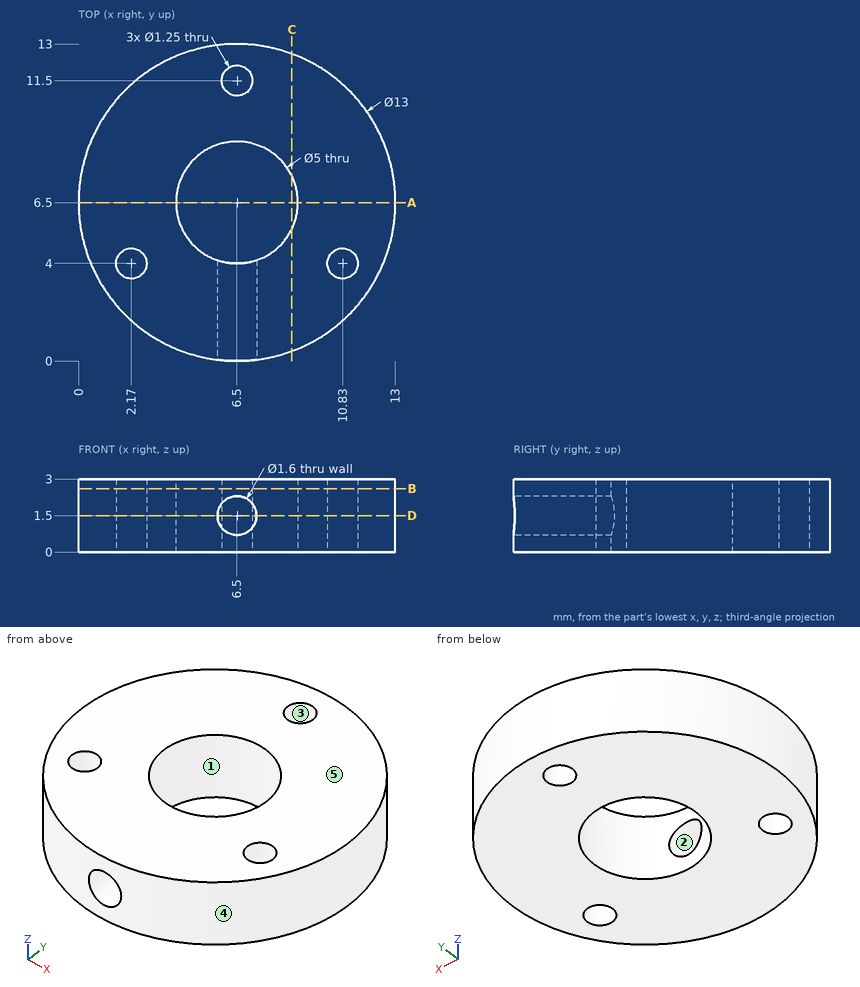
The figure shows three views and two pictorial views of one solid part (mm, origin at its lowest corner). Answer the questions. A direction names the side the tool comes from. Coordinates: 2 decimals unless noted, no trailing zeros. Order: outer loops, then holes, each group sorted by start corner. A loop starts at its lowest first (then second) coordinate and runs counter-clockwise, first axis right, second up.
Q1. Which of the six approach directions +Z, -Z, +X, -X, +Y, -Y give full straight-line access (tool end or side, diameter ignored) to the marked faces 1 and 2?
Q2. A cutting plane is placed at C-C, the plane x = 8.75. Write down the section's boundary in (y, z).
Q3. A cutting plane is placed at D-D, the plane z = 1.5. State how many separate pieces and enclosed holes the cut face has, and give its area (3 significant figures).
Q4. For a pull along X with two mould halves and no side action, classify the marked faces 3, 4 and 5 as pulls with the +X half, pulls with the -X half, needs draft (parallel to the pull), parting line crosses it, or undercut.
Q5. A cutting plane is placed at A-A, the plane y = 6.5. Write down the section's boundary in (x, z), and give its area (3 significant figures).
Q6. Consider line 1 (Y direction, x = 6.5, z = 0.8) (3 decimals); line 2 (X direction, y = 3.75, z = 1.7) (1 decimal); line 3 (X direction, y = 3.5, z = 0.45) (1 decimal). Determine where each line is inside the solid, lowest interval first.
Q7. A cutting plane is placed at B-B, the plane z = 2.6. Write down the section's boundary in (x, y) (3 decimals).
Answers follow:
1. face 1: +Z, -Z
1. face 2: -Y
2. outline: (0.4, 0) - (5.41, 0) - (5.41, 3) - (0.4, 3) - close; (7.59, 0) - (12.6, 0) - (12.6, 3) - (7.59, 3) - close
3. separate pieces: 1
3. enclosed holes: 3
3. area: 103 mm2
4. face 3: undercut
4. face 4: parting line crosses it
4. face 5: needs draft
5. outline: (0, 0) - (4, 0) - (4, 3) - (0, 3) - close; (9, 0) - (13, 0) - (13, 3) - (9, 3) - close
5. area: 24.0 mm2
6. line 1: y = 9 to 10.875, 12.125 to 13
6. line 2: x = 0.6 to 1.6, 2.7 to 5.7, 7.3 to 10.3, 11.4 to 12.4
6. line 3: x = 0.7 to 1.8, 2.5 to 10.5, 11.2 to 12.3
7. outline: circle Ø13 at (6.5, 6.5); hole circle Ø1.25 at (2.17, 4); hole circle Ø5 at (6.5, 6.5); hole circle Ø1.25 at (6.5, 11.5); hole circle Ø1.25 at (10.83, 4)
